from build123d import *

# Parameters (mm, degrees)
SKETCH1_R           = 12.5
SKETCH1_R_2         = 1.5
SKETCH1_R_3         = 2.5
BOSS_EXTRUDE1_DEPTH = 6
FILLET1_R           = 10
SKETCH2_R           = 1.5
SKETCH2_R_2         = 30
CUT_EXTRUDE1_DEPTH  = 10


with BuildPart() as part:
    # Sketch1 → Boss-Extrude1 (new body)
    with BuildSketch(Plane.XY):
        Polygon((-145, 120), (145, 120), (145, -8.284271247), (0, -153.284271247), (-145, -8.284271247), align=None)
        with Locations((0, -125)):
            Circle(SKETCH1_R, mode=Mode.SUBTRACT)
        with Locations((-137.374368671, 87.625631329)):
            Circle(SKETCH1_R_2, mode=Mode.SUBTRACT)
        with Locations((-112.625631329, 112.374368671)):
            Circle(SKETCH1_R_2, mode=Mode.SUBTRACT)
        with Locations((-137.374368671, 12.374368671)):
            Circle(SKETCH1_R_2, mode=Mode.SUBTRACT)
        with Locations((-125, -17.5)):
            Circle(SKETCH1_R_2, mode=Mode.SUBTRACT)
        with Locations((-17.5, -125)):
            Circle(SKETCH1_R_2, mode=Mode.SUBTRACT)
        with Locations(Location((17.5, -125, 0), (0, 0, 180))):
            Circle(SKETCH1_R_2, mode=Mode.SUBTRACT)
        with Locations(Location((125, -17.5, 0), (0, 0, 180))):
            Circle(SKETCH1_R_2, mode=Mode.SUBTRACT)
        with Locations(Location((137.374368671, 12.374368671, 0), (0, 0, 180))):
            Circle(SKETCH1_R_2, mode=Mode.SUBTRACT)
        with Locations(Location((137.374368671, 87.625631329, 0), (0, 0, 180))):
            Circle(SKETCH1_R_2, mode=Mode.SUBTRACT)
        with Locations(Location((112.625631329, 112.374368671, 0), (0, 0, 180))):
            Circle(SKETCH1_R_2, mode=Mode.SUBTRACT)
        with Locations((0, 100)):
            Circle(SKETCH1_R_3, mode=Mode.SUBTRACT)
        with Locations((-125, 100)):
            Circle(SKETCH1_R_3, mode=Mode.SUBTRACT)
        with Locations((125, 100)):
            Circle(SKETCH1_R_3, mode=Mode.SUBTRACT)
        Circle(SKETCH1_R_3, mode=Mode.SUBTRACT)
    extrude(amount=BOSS_EXTRUDE1_DEPTH)

    # Fillet1
    fillet1_edges = [part.edges().sort_by_distance(p)[0] for p in [
        (145, -8.284271247, 3),
        (0, -153.284271247, 3),
        (-145, -8.284271247, 3),
    ]]
    fillet(fillet1_edges, radius=FILLET1_R)

    # Sketch2 → Cut-Extrude1 (cut)
    with BuildSketch(Plane.XY.offset(6)):
        with Locations((38.67402397, 24.920368197)):
            Circle(SKETCH2_R)
        with Locations((89.920368197, 56.32597603)):
            Circle(SKETCH2_R)
        with Locations((121.32597603, 5.079631803)):
            Circle(SKETCH2_R)
        with Locations((70.079631803, -26.32597603)):
            Circle(SKETCH2_R)
        with Locations((80, 15)):
            Circle(SKETCH2_R_2)
        with Locations(Location((-38.67402397, 24.920368197, 0), (0, 0, 180))):
            Circle(SKETCH2_R)
        with Locations(Location((-89.920368197, 56.32597603, 0), (0, 0, 180))):
            Circle(SKETCH2_R)
        with Locations(Location((-70.079631803, -26.32597603, 0), (0, 0, 180))):
            Circle(SKETCH2_R)
        with Locations(Location((-121.32597603, 5.079631803, 0), (0, 0, 180))):
            Circle(SKETCH2_R)
        with Locations(Location((-80, 15, 0), (0, 0, 180))):
            Circle(SKETCH2_R_2)
    extrude(amount=-CUT_EXTRUDE1_DEPTH, mode=Mode.SUBTRACT)


solid = part.part
The listing builds one solid part. Answer for the finished solid, in the listing's coordinates (mm). Coordinates: 2 decimals unless noted, no trailing zeros. Loops run counter-clockwise (first coordinate to the right, second up) from the corner with the lowest first, then second, coordinate; pieces in that order, holes last.
1) Find the intervals of material crossed by L1, parallel to X at y = 36.5, z = 2.55; L2, parallel to X at y = 102, z = 3.4; L3, parallel to X at y = 30, z = 4.9, in increasing order.
2) Flat-ended cylindrical pins translate along their axes: pin 1 Ø2 at (y, z) = (-118, 3) entering from +X; pin 2 Ø1.5 at (y, z) = (-103.5, 4) entering from +X; pin 3 Ø1 at (y, z) = (-111.5, 5.5) entering from +X. Find the tip coordinate at first contact, or state that the pin passes through.
3) Find section C-C on x = -95.5. Write down the section's boundary in (y, z).
4) Find section B-B on z = 2.1. Give the number of separate pieces and of enclosed holes in the cut face, then the cut area to 3 significant figures.
5) Find section A-A on x = 97.5. Write down the section's boundary in (y, z), then the cut area to 3 significant figures.
6) Determine the mould class of faces 1 (the face through (50.03, 16.32, 3.04)), 2 (the face through (145, 59, 3)), 3 (the face through (-73.626, -79.658, 2.958)) for opening direction X: pulls with the +X half, pulls with the -X half, needs draft (parallel to the pull), parting line crosses it, or undercut.
7) Find section D-D on y = -79. Write down the section's boundary in (x, z), then the cut area to 3 significant figures.
Values:
1. L1: x = -145 to -100.92, -59.08 to 59.08, 100.92 to 145
1. L2: x = -145 to -126.5, -123.5 to -1.5, 1.5 to 123.5, 126.5 to 145
1. L3: x = -145 to -105.98, -54.02 to 54.02, 105.98 to 145
2. pin 1: stops at x = 36.28
2. pin 2: stops at x = 50.53
2. pin 3: stops at x = 42.28
3. outline: (-57.78, 0) - (-10.69, 0) - (-10.69, 6) - (-57.78, 6) - close; (40.69, 0) - (120, 0) - (120, 6) - (40.69, 6) - close
4. separate pieces: 1
4. enclosed holes: 25
4. area: 51,900 mm2
5. outline: (-55.78, 0) - (-9.37, 0) - (-9.37, 6) - (-55.78, 6) - close; (39.37, 0) - (120, 0) - (120, 6) - (39.37, 6) - close
5. area: 762 mm2
6. face 1: undercut
6. face 2: pulls with the +X half
6. face 3: pulls with the -X half
7. outline: (-74.28, 0) - (74.28, 0) - (74.28, 6) - (-74.28, 6) - close
7. area: 891 mm2
